Read the model definition and answer for the solid it produces. Units are mm, in the model's axes. Face numbers are marked on the shaded views. A direction names the side the tool comes from. Give positions to 0.01 mm unless a question says otherwise; leave off trailing zeros. Write each loop counter-clockwise with the first axis right and the second up, starting at its lowest first coordinate (ties: lowest second). Pieces come first, ordered by that corner, then holes. Notation, with made-up numbers: (34, 7.5) -> (46, 7.5) arc R29 cw to (46, 37.5) -> close; hole circle Ø5 at (-6.75, 52). An arc over 180 degrees is marked (long way). Write item = value, one per line.
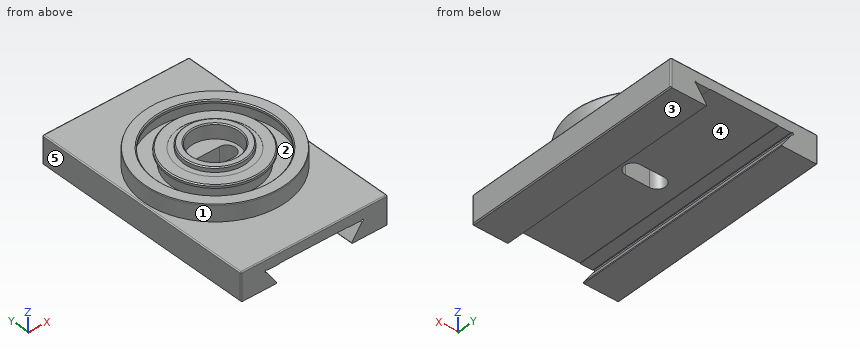
from build123d import *
from OCP.BRepFilletAPI import BRepFilletAPI_MakeChamfer

# Parameters (mm, degrees)
BOSS_EXTRUDE1_DEPTH = 147.6375
CUT_EXTRUDE1_DEPTH  = 313.398864885
SKETCH2_R           = 92.075
BOSS_EXTRUDE2_DEPTH = 21.4875
SKETCH5_R           = 40
BOSS_EXTRUDE3_DEPTH = 6
CUT_EXTRUDE4_START  = -0.254
SKETCH8_R           = 46.99
SKETCH8_R_2         = 40
CUT_EXTRUDE4_DEPTH  = 0.254
SKETCH6_R           = 31
CUT_EXTRUDE2_DEPTH  = 19
CUT_EXTRUDE3_DEPTH  = 38.1
CHAMFER3_SIZE       = 1.27
CHAMFER1_SIZE       = 1.27
CHAMFER1_SIZE2      = 1.329072894
FILLET1_R           = 1.27
CHAMFER2_SIZE       = 1.27
CHAMFER2_SIZE2      = 0.462242198
CHAMFER4_SIZE       = 1.27


with BuildPart() as part:
    # Sketch1 → Boss-Extrude1 (new, symmetric)
    with BuildSketch(Plane(origin=(0, 0, 0), x_dir=(1, 0, 0), z_dir=(0, 1, 0))):
        Polygon((-95.25, 36.5125), (-95.25, 0), (95.25, 0), (95.25, 36.5125), (47.937887463, 36.5125), (63.5, 14.2875), (44.45, 14.2875), (44.45, 13.6525), (-44.45, 13.6525), (-44.45, 14.2875), (-63.5, 14.2875), (-47.937887463, 36.5125), align=None)
    extrude(amount=BOSS_EXTRUDE1_DEPTH, both=True)

    # Sketch3 → Cut-Extrude1 (cut, through all)
    with BuildSketch(Plane(origin=(0, 147.6375, 0), x_dir=(1, 0, 0), z_dir=(0, 1, 0))):
        Polygon((-61.922427153, 16.540507516), (-64.17543467, 15.367666039), (-63.002593192, 13.114658522), (-60.749585676, 14.2875), align=None)
        Polygon((64.17543467, 15.367666039), (61.922427153, 16.540507516), (60.749585676, 14.2875), (63.002593192, 13.114658522), align=None)
    extrude(amount=-CUT_EXTRUDE1_DEPTH, mode=Mode.SUBTRACT)

    # Sketch2 → Boss-Extrude2 (add)
    with BuildSketch(Plane.XY):
        with Locations(Location((0, 0, 0), (0, 0, 180))):
            Circle(SKETCH2_R)
    extrude(amount=BOSS_EXTRUDE2_DEPTH)

    # Sketch4 → Cut-Revolve1 (revolve, cut)
    with BuildSketch(Plane(origin=(0, 0, 0), x_dir=(0, 0, -1), z_dir=(1, 0, 0))):
        Polygon((-28.064444951, 76.96), (-17.564444869, 76.96), (-17.564444869, 81.46), (-2.064444951, 81.46), (-2.064444951, 56.46), (-17.564444869, 56.46), (-17.564444869, 60.96), (-28.064444951, 60.96), align=None)
    revolve(axis=Axis((0, 0, 0), (0, 0, 1)), mode=Mode.SUBTRACT)

    # Sketch5 → Boss-Extrude3 (add)
    with BuildSketch(Plane.XY.offset(21.4875)):
        Circle(SKETCH5_R)
    extrude(amount=BOSS_EXTRUDE3_DEPTH)

    # Sketch8 → Cut-Extrude4 (cut)
    with BuildSketch(Plane.XY.offset(21.4875).offset(CUT_EXTRUDE4_START)):
        Circle(SKETCH8_R)
        Circle(SKETCH8_R_2, mode=Mode.SUBTRACT)
    extrude(amount=CUT_EXTRUDE4_DEPTH, mode=Mode.SUBTRACT)

    # Sketch6 → Cut-Extrude2 (cut)
    with BuildSketch(Plane.XY.offset(27.4875)):
        Circle(SKETCH6_R)
    extrude(amount=-CUT_EXTRUDE2_DEPTH, mode=Mode.SUBTRACT)

    # Sketch7 → Cut-Extrude3 (cut)
    with BuildSketch(Plane.XY.offset(8.4875)):
        with BuildLine():
            Line((15.45, -11.05), (-15.45, -11.05))
            ThreePointArc((-15.45, -11.05), (-26.5, 0), (-15.45, 11.05))
            Line((-15.45, 11.05), (15.45, 11.05))
            ThreePointArc((15.45, 11.05), (26.5, 0), (15.45, -11.05))
        make_face()
    extrude(amount=-CUT_EXTRUDE3_DEPTH, mode=Mode.SUBTRACT)

    # Chamfer3
    chamfer3_edges = [part.edges().sort_by_distance(p)[0] for p in [
        (95.25, 0, -36.5125),
        (-95.25, 0, -36.5125),
    ]]
    chamfer(chamfer3_edges, length=CHAMFER3_SIZE)

    # Chamfer1: one chamfer whose edges measure the first distance from different faces: ONE call of the kernel's chamfer builder (chamfer() names one face for all edges)
    chamfer1_edges_1 = [part.edges().sort_by_distance(p)[0] for p in [
        (47.937887463, 0, -36.5125),
    ]]
    chamfer1_side_1 = [part.faces().sort_by_distance(p)[0] for p in [
        (54.930157308, 0, -26.526503758),
    ]]
    chamfer1_edges_2 = [part.edges().sort_by_distance(p)[0] for p in [
        (-47.937887463, 0, -36.5125),
    ]]
    chamfer1_side_2 = [part.faces().sort_by_distance(p)[0] for p in [
        (-70.958943732, 0, -36.5125),
    ]]
    chamfer1 = BRepFilletAPI_MakeChamfer(part.part.solid().wrapped)
    for e in chamfer1_edges_1:
        chamfer1.Add(CHAMFER1_SIZE, CHAMFER1_SIZE2, e.wrapped, chamfer1_side_1[0].wrapped)  # the first distance lies on this face
    for e in chamfer1_edges_2:
        chamfer1.Add(CHAMFER1_SIZE, CHAMFER1_SIZE2, e.wrapped, chamfer1_side_2[0].wrapped)  # the first distance lies on this face
    add(Compound.cast(chamfer1.Shape()), mode=Mode.REPLACE)

    # Fillet1
    fillet1_edges = [part.edges().sort_by_distance(p)[0] for p in [
        (95.25, -147.6375, -17.62125),
        (-95.25, -147.6375, -17.62125),
        (0, -147.6375, 0),
        (95.25, 0, 0),
        (95.25, 147.6375, -17.62125),
        (-95.25, 147.6375, -17.62125),
        (0, 147.6375, 0),
        (-95.25, 0, 0),
    ]]
    fillet(fillet1_edges, radius=FILLET1_R)

    # Chamfer2
    chamfer2_edges = [part.edges().sort_by_distance(p)[0] for p in [
        (92.075, 0, 21.4875),
    ]]
    chamfer2_side = [part.faces().sort_by_distance(p)[0] for p in [
        (92.075, 0, 10.74375),
    ]]
    chamfer(chamfer2_edges, length=CHAMFER2_SIZE, length2=CHAMFER2_SIZE2, reference=chamfer2_side[0])

    # Chamfer4
    chamfer4_edges = [part.edges().sort_by_distance(p)[0] for p in [
        (0, -76.96, 21.4875),
        (0, -60.96, 21.4875),
        (-40, 0, 27.4875),
        (-31, 0, 27.4875),
    ]]
    chamfer(chamfer4_edges, length=CHAMFER4_SIZE)


solid = part.part
(1) A tool of negligible diameter and unlimited length cuts with its end or side. For the marked faces 4 and 5, from which of +Z, -Z, +X, -X, +Y, -Y can it reach the whole face along a straight path? Write none if from no direction.
Checks:
face_4 = -Z, +Y, -Y
face_5 = +Z, -Z, -X, +Y, -Y
(2) Given P1, Ø1.5, axis at y = -44.5, z = 15, coming from the +X side; P2, Ø4, axis at x = 48.5, z = -15, coming from the +Y side; P3, Ø5, axis at x = -65.5, y = 83, coming from the +Z side; P4, Ø2, axis at x = 32, y = -106.5, coming from the -Z side, each flat-ended and moving along its own axis, determine where each tip first touches the part or whether it passes through.
Checks:
P1 = 81.02
P2 = 147.64
P3 = 0
P4 = -13.65
(3) Consider L1, parallel to Y at x = 0, z = 16 (3 decimals); L2, parallel to Y at x = 0, z = 22; L3, parallel to Y at x = 20.5, z = 19.5. Determine where each line is inside the solid, lowest interval first.
Checks:
L1 = -92.075 to -81.46, -56.46 to -31, 31 to 56.46, 81.46 to 92.075
L2 = -40 to -31, 31 to 40
L3 = -89.76 to -74.18, -57.41 to -23.25, 23.25 to 57.41, 74.18 to 89.76
(4) For a pull along X with two mould halves and no side action, classify the marked faces 1, 2 and 3 as released by +X, released by -X, zero draft, split by the parting line, or undercut.
Checks:
face_1 = split by the parting line
face_2 = undercut
face_3 = zero draft
(5) The part is cut by section B-B on y = 119.5. Determine the outline of the cut face in (x, z), plus the area to 3 significant figures.
Checks:
outline = (-95.25, -35.24) -> (-93.98, -36.51) -> (-49.21, -36.51) -> (-48.7, -35.42) -> (-61.92, -16.54) -> (-64.18, -15.37) -> (-63, -13.11) -> (-60.75, -14.29) -> (-44.45, -14.29) -> (-44.45, -13.65) -> (44.45, -13.65) -> (44.45, -14.29) -> (60.75, -14.29) -> (63, -13.11) -> (64.18, -15.37) -> (61.92, -16.54) -> (48.67, -35.47) -> (49.27, -36.51) -> (93.98, -36.51) -> (95.25, -35.24) -> (95.25, -1.27) arc R1.27 ccw to (93.98, 0) -> (-93.98, 0) arc R1.27 ccw to (-95.25, -1.27) -> close
area = 4,410 mm²
(6) The part is cut by section A-A on z = -24.5. Determine the outline of the cut face in (x, y), plus the area to 3 significant figures.
Checks:
outline = (-95.25, -146.37) arc R1.27 ccw to (-93.98, -147.64) -> (-56.35, -147.64) -> (-56.35, 147.64) -> (-93.98, 147.64) arc R1.27 ccw to (-95.25, 146.37) -> close; (56.35, -147.64) -> (93.98, -147.64) arc R1.27 ccw to (95.25, -146.37) -> (95.25, 146.37) arc R1.27 ccw to (93.98, 147.64) -> (56.35, 147.64) -> close
area = 23,000 mm²
